Geometry check sheet. Reference: the model listing, model coordinates, mm. Face numbers are marked on the shaded views. A direction names the side the tool comes from. Round coordinates to 2 decimals unless told otherwise and drop trailing zeros. Write each loop counter-clockwise with the first axis right and the second up, starting at its lowest first coordinate (ties: lowest second). Pieces come first, ordered by that corner, then holes. Notation, with made-up numbers: M -31,66.5 L -20,66.5 A26 ccw -20,95.5 Z; hole C -6,0.25 d6. An arc over 180 degrees is marked long. One line per item, written item: value. Start each with the question number.
1. Section check A-A (y = 0). Record the boundary of the cut face in (x, z), and give its area (3 significant figures).
2. Scan lines: probe 1 along X at (y, z) = (8.5, -7.75); probe 2 along Z at (x, y) = (-7.25, -0.5); probe 3 along X at (y, z) = (-5, -3.25). Record each from-to range of solid material in increasing order. Write a range as [from, to].
3. Section check C-C (x = 11). Record the boundary of the cut face in (y, z), and give its area (3 significant figures).
4. Access from +Z, -Z, +X, -X, +Y, -Y to the whole of each face (thin tool, end or side, straight path). Record for the marked faces 5 and 6.
5. Release check for a two-part mould opening along X. For the marked faces 1, 2, 3 and 4 record: pulls with the +X half, pulls with the -X half, needs draft (parallel to the pull), parting line crosses it, or undercut.
6. Section check D-D (x = 3). Record the boundary of the cut face in (y, z), and give its area (3 significant figures).
7. Depth check by flat-ended pin: P1, Ø8, axis at x = -9.5, y = -5.5, coming from the -Z side; P2, Ø1.5, axis at x = -9.5, y = 11.5, coming from the -Z side; P3, Ø6, axis at x = -7, y = -3.5, coming from the +Z side. Enter the tip coordinate at first touch or a pass-through.
from build123d import *

# Parameters (mm, degrees)
SKETCH1_R           = 15
BOSS_EXTRUDE1_DEPTH = 15


with BuildPart() as part:
    # Sketch1 → Boss-Extrude1 (new, symmetric)
    with BuildSketch(Plane(origin=(0, 0, 0), x_dir=(0, 0, -1), z_dir=(1, 0, 0))):
        Circle(SKETCH1_R)
    extrude(amount=BOSS_EXTRUDE1_DEPTH, both=True)

    # Sketch2 → Cut-Revolve1 (revolve, cut)
    with BuildSketch(Plane.XY, mode=Mode.PRIVATE) as cut_revolve1_sk:
        Polygon((-5, 15), (5, 15), (2.5, 5), (-2.5, 5), align=None)
    revolve(cut_revolve1_sk.sketch.rotate(Axis((0, 0, 0), (1, 0, 0)), 90), axis=Axis((0, 0, 0), (1, 0, 0)), mode=Mode.SUBTRACT)


solid = part.part
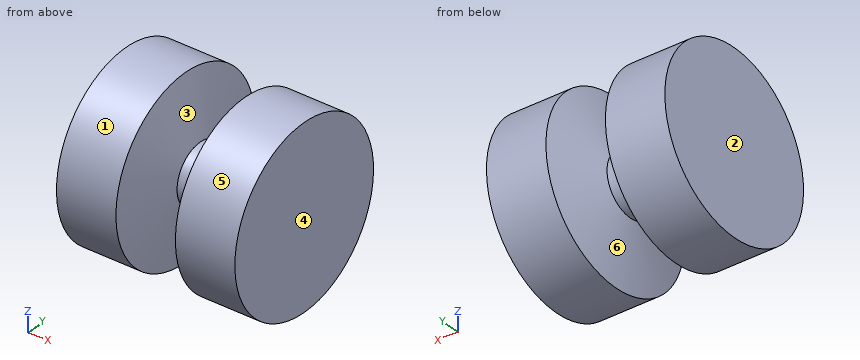
Result sheet:
1. outline: M -15,-15 L -5,-15 L -2.5,-5 L 2.5,-5 L 5,-15 L 15,-15 L 15,15 L 5,15 L 2.5,5 L -2.5,5 L -5,15 L -15,15 Z
1. area: 750 mm2
2. probe 1: x = [-15, -4.13], [4.13, 15]
2. probe 2: z = [-14.99, 14.99]
2. probe 3: x = [-15, -2.74], [2.74, 15]
3. outline: C 0,0 d30
3. area: 707 mm2
4. face 5: +X, -X
4. face 6: none
5. face 1: needs draft
5. face 2: pulls with the -X half
5. face 3: undercut
5. face 4: pulls with the +X half
6. outline: C 0,0 d14
6. area: 154 mm2
7. P1: stops at z = -14.92
7. P2: stops at z = -10.46
7. P3: stops at z = 14.99
